```python
from build123d import *

# Parameters (mm, degrees)
F0_W     = 101.6
F0_H     = 48.26
F1_DEPTH = 114.3
F3_DEPTH = 177.8
F4_R     = 4.7625
F5_DEPTH = 25.4


with BuildPart() as f1:
    # F0 (on Top) → F1 (new body, symmetric)
    with BuildSketch(Plane.XY):
        Rectangle(F0_W, F0_H)
    extrude(amount=F1_DEPTH, both=True)

    # F2 (on face) → F3 (cut)
    with BuildSketch(Plane(origin=(0, 0, -114.3), x_dir=(1, 0, 0), z_dir=(0, 0, -1))):
        Polygon((30.48, 24.13), (-30.48, 24.13), (-30.48, 3.81), (-50.8, 3.81), (-50.8, -3.81), (-30.48, -3.81), (-30.48, -24.13), (30.48, -24.13), (30.48, -3.81), (50.8, -3.81), (50.8, 3.81), (30.48, 3.81), align=None)
    extrude(amount=-F3_DEPTH, mode=Mode.SUBTRACT)

    # F4 (on face) → F5 (cut)
    with BuildSketch(Plane.XY.offset(114.3)):
        Circle(F4_R)
    extrude(amount=-F5_DEPTH, mode=Mode.SUBTRACT)


solid = f1.part
```
For this review, take the finished solid that the model builds, in its own axes (mm). A direction names the side the tool comes from. Round coordinates to 2 decimals unless told otherwise and drop trailing zeros. Order: outer loops, then holes, each group sorted by start corner. A loop starts at its lowest first (then second) coordinate and runs counter-clockwise, first axis right, second up.
Q1. Mouldability with a two-part tool opening along X and no side actions: class faces 1 (the flat face through (50.8, 5, 2)), 2 (the flat face through (-30.48, 14, -27)), 3 (the flat face through (40, 14, -114.3)) as pulls with the +X half, pulls with the -X half, needs draft (parallel to the pull), parting line crosses it, or undercut.
Findings below:
face 1: pulls with the +X half
face 2: undercut
face 3: needs draft
Q2. We need section C-C, the plane x = 0. Give the boundary of the cut face in (y, z), plus the area to 3 significant figures.
Findings below:
outline: (-24.13, 63.5) - (24.13, 63.5) - (24.13, 114.3) - (4.76, 114.3) - (4.76, 88.9) - (-4.76, 88.9) - (-4.76, 114.3) - (-24.13, 114.3) - close
area: 2,210 mm2
Q3. We need section D-D, the plane x = 18.5. Give the boundary of the cut face in (y, z), plus the area to 3 significant figures.
Findings below:
outline: (-24.13, 63.5) - (24.13, 63.5) - (24.13, 114.3) - (-24.13, 114.3) - close
area: 2,450 mm2
Q4. We need section B-B, the plane y = 0. Give the boundary of the cut face in (x, z).
Findings below:
outline: (-50.8, 63.5) - (50.8, 63.5) - (50.8, 114.3) - (4.76, 114.3) - (4.76, 88.9) - (-4.76, 88.9) - (-4.76, 114.3) - (-50.8, 114.3) - close
Q5. We need section A-A, the plane z = 21. Give the boundary of the cut face in (x, y).
Findings below:
outline: (-50.8, -24.13) - (-30.48, -24.13) - (-30.48, -3.81) - (-50.8, -3.81) - close; (-50.8, 3.81) - (-30.48, 3.81) - (-30.48, 24.13) - (-50.8, 24.13) - close; (30.48, -24.13) - (50.8, -24.13) - (50.8, -3.81) - (30.48, -3.81) - close; (30.48, 3.81) - (50.8, 3.81) - (50.8, 24.13) - (30.48, 24.13) - close
Q6. Machinability: for faces 4 (the flat face through (-41, -14, -114.3)), 5 (the flat face through (-41, 3.81, -27)), 6 (the flat face through (0, 0, 88.9)), 7 (the flat face through (30.48, -14, -27)), 8 (the flat face through (-1, 6, 114.3)), which of the approach directions +Z, -Z, +X, -X, +Y, -Y give a long, thin tool a straight path to every point of the face, cutting with its end or side? Answer none if there is none.
Findings below:
face 4: -Z, +X, -X, +Y, -Y
face 5: -Z, +X, -X
face 6: +Z
face 7: -Z, +Y, -Y
face 8: +Z, +X, -X, +Y, -Y
Q7. Insertion check: P1, Ø8, axis at x = 10.5, y = 15, coming from the -Z side; P2, Ø3, axis at x = -2, y = 2, coming from the +Z side. Each pin has a flat end and moves straight along its axis. Give the tip position at first contact, or say it passes through.
Findings below:
P1: stops at z = 63.5
P2: stops at z = 88.9
Q8. Wall thickness on line 1 (X direction, y = -13, z = 63); line 2 (Y direction, x = -33, z = -42.5); line 3 (Y direction, x = 0, z = 106): over which ranges is each line inside the solid? List them lowest first.
Findings below:
line 1: x = -50.8 to -30.48, 30.48 to 50.8
line 2: y = -24.13 to -3.81, 3.81 to 24.13
line 3: y = -24.13 to -4.76, 4.76 to 24.13
